Could you check a few things on this model? Use its own coordinates, in mm. Face numbers are marked on the shaded views. A direction names the side the tool comes from. Round coordinates to 2 decimals unless told otherwise and drop trailing zeros. Loops run counter-clockwise (first coordinate to the right, second up) from the corner with the lowest first, then second, coordinate; pieces in that order, holes last. Notation, with made-up numbers: (-35.75, 42.5) -> (-12.75, 42.5) arc R24 ccw to (-12.75, 80.5) -> close; hole circle Ø1 at (41, 33.5). An arc over 180 degrees is marked (long way). Put each result on its own line as item: value. Start each with the question number.
1. Imagine slicing it at A-A, the plane x = 756. Please give me the cut outline in (y, z), and give its area (3 significant figures).
2. I need wall thicknesses on line 1 (Z direction, x = 756, y = 562.5); line 2 (Z direction, x = 755.5, y = 558); line 3 (X direction, y = 556, z = 17). Which ranges of each line are inside material? Lowest first, please. Write a range as [from, to].
3. I'm going to push flat-ended pins straight in: P1, Ø0.9, axis at x = 756, z = 45, coming from the +Y side; P2, Ø0.9, axis at x = 756, z = 2.5, coming from the -Y side; P3, Ø2, axis at x = 757, z = 20.5, coming from the -Y side; P4, Ø4, axis at y = 560.3, z = 36.37, coming from the +X side. Where does each tip first touch, or does it pass through?
4. Imagine slicing it at C-C, the plane x = 760.5. Please give me the cut outline in (y, z), and give its area (3 significant figures).
5. Imagine slicing it at B-B, the plane z = 16. Please give me the cut outline in (x, y).
6. Which directions (+Z, -Z, +X, -X, +Y, -Y) give clear straight access to the entire face, cutting with the end or side of a thin tool? Please do the marked faces 1, 2 and 3.
7. Imagine slicing it at D-D, the plane y = 561.5. Count the separate pieces of the cut face and the enclosed holes in it, and give its area (3 significant figures).
```python
from build123d import *

# Parameters (mm, degrees)
EXTRUDE1_DEPTH                            = 47.371
SKETCH2_R                                 = 1.3843
CUT_EXTRUDE1_DEPTH                        = 7.35
CSK_FOR_8_FLAT_HEAD_MACHINE_SCREW_2_COUNT = 2
CSK_FOR_8_FLAT_HEAD_MACHINE_SCREW_2_PITCH = 25.4


with BuildPart() as part:
    # Sketch1 → Extrude1 (new body)
    with BuildSketch(Plane.XY):
        with BuildLine():
            Line((761.528249985, 570.229723122), (761.528249985, 550.366923122))
            ThreePointArc((761.528249985, 550.366923122), (761.416657669, 550.097515438), (761.147249985, 549.985923122))
            Line((761.147249985, 549.985923122), (758.099249985, 549.985923122))
            ThreePointArc((758.099249985, 549.985923122), (757.829842301, 550.097515438), (757.718249985, 550.366923122))
            Line((757.718249985, 550.366923122), (757.718249985, 556.742323122))
            ThreePointArc((757.718249985, 556.742323122), (757.606657669, 557.011730805), (757.337249985, 557.123323122))
            Line((757.337249985, 557.123323122), (755.559249985, 557.123323122))
            ThreePointArc((755.559249985, 557.123323122), (755.289842301, 557.234915438), (755.178249985, 557.504323122))
            Line((755.178249985, 557.504323122), (755.178249985, 563.092323122))
            ThreePointArc((755.178249985, 563.092323122), (755.289842301, 563.361730805), (755.559249985, 563.473323122))
            Line((755.559249985, 563.473323122), (757.337249985, 563.473323122))
            ThreePointArc((757.337249985, 563.473323122), (757.606657669, 563.584915438), (757.718249985, 563.854323122))
            Line((757.718249985, 563.854323122), (757.718249985, 570.229723122))
            ThreePointArc((757.718249985, 570.229723122), (757.829842301, 570.499130805), (758.099249985, 570.610723122))
            Line((758.099249985, 570.610723122), (761.147249985, 570.610723122))
            ThreePointArc((761.147249985, 570.610723122), (761.416657669, 570.499130805), (761.528249985, 570.229723122))
        make_face()
    extrude(amount=EXTRUDE1_DEPTH)

    # Sketch2 → Cut-Extrude1 (cut, through all)
    with BuildSketch(Plane.ZY.offset(-755.178249985)):
        with Locations((10.9728, 560.298323122)):
            Circle(SKETCH2_R)
        with Locations((36.3728, 560.298323122)):
            Circle(SKETCH2_R)
    extrude(amount=-CUT_EXTRUDE1_DEPTH, mode=Mode.SUBTRACT)

    # Sketch3 → CSK for #8 Flat Head Machine Screw (100)1 (revolve, cut)
    with BuildSketch(Plane(origin=(755.178249985, 560.298323122, 10.9728), x_dir=(0, 0, 1), z_dir=(0, 1, 0))):
        Polygon((0, 0), (0, 6.35), (2.2479, 6.35), (2.2479, 3.886967624), (4.2164, 2.2352), (4.2164, 0), align=None)
    csk_for_8_flat_head_machine_screw_100 = revolve(axis=Axis((748.828249985, 560.298323122, 10.9728), (1, 0, 0)), mode=Mode.SUBTRACT)

    # CSK for _8 Flat Head Machine Screw _ 2: CSK for #8 Flat Head Machine Screw (100)1 ×2
    with Locations(*[(0, 0, i * CSK_FOR_8_FLAT_HEAD_MACHINE_SCREW_2_PITCH) for i in range(1, CSK_FOR_8_FLAT_HEAD_MACHINE_SCREW_2_COUNT)]):
        add(csk_for_8_flat_head_machine_screw_100, mode=Mode.SUBTRACT)


solid = part.part
```
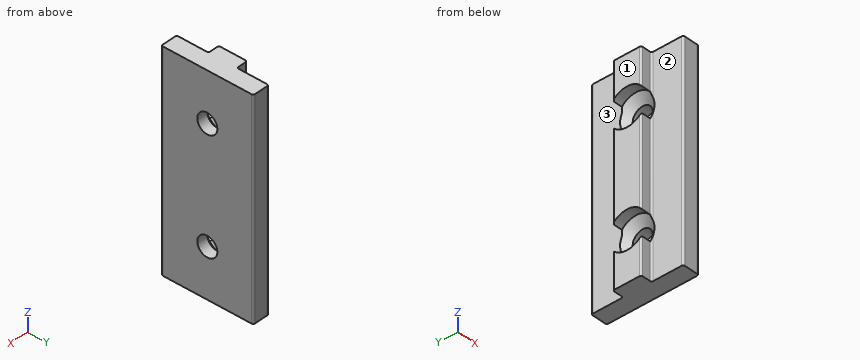
Entries:
1. outline: (557.12, 0) -> (563.47, 0) -> (563.47, 8.2) arc R4.22 cw to (557.12, 8.2) -> close; (557.12, 13.75) arc R4.22 cw to (563.47, 13.75) -> (563.47, 33.6) arc R4.22 cw to (557.12, 33.6) -> close; (557.12, 39.15) arc R4.22 cw to (563.47, 39.15) -> (563.47, 47.37) -> (557.12, 47.37) -> close
1. area: 205 mm^2
2. line 1: [0, 7.38], [14.57, 32.78], [39.97, 47.37]
2. line 2: [0, 7.44], [14.51, 32.84], [39.91, 47.37]
2. line 3: [757.72, 761.53]
3. P1: y = 563.47
3. P2: y = 557.12
3. P3: y = 550
3. P4: through
4. outline: (549.99, 0) -> (570.61, 0) -> (570.61, 47.37) -> (549.99, 47.37) -> close; hole circle Ø4.5 at (560.3, 10.97); hole circle Ø4.5 at (560.3, 36.37)
4. area: 945 mm^2
5. outline: (755.18, 557.5) arc R0.38 ccw to (755.56, 557.12) -> (757.34, 557.12) arc R0.38 cw to (757.72, 556.74) -> (757.72, 550.37) arc R0.38 ccw to (758.1, 549.99) -> (761.15, 549.99) arc R0.38 ccw to (761.53, 550.37) -> (761.53, 570.23) arc R0.38 ccw to (761.15, 570.61) -> (758.1, 570.61) arc R0.38 ccw to (757.72, 570.23) -> (757.72, 563.85) arc R0.38 cw to (757.34, 563.47) -> (755.56, 563.47) arc R0.38 ccw to (755.18, 563.09) -> close
6. face 1: +Z, -Z, -X, +Y, -Y
6. face 2: +Z, -Z, -X, -Y
6. face 3: +Z, -Z, -X, +Y
7. separate pieces: 3
7. enclosed holes: 0
7. area: 226 mm^2
